Print and shaded views of the part. All mm, measured from the part's lowest x, y and z. A direction names the side the tool comes from. Coordinates: 2 decimals unless noted, no trailing zeros. Order: outer loops, then holes, each group sorted by start corner. A loop starts at its lowest first (then second) coordinate and runs counter-clockwise, first axis right, second up. Notation, with made-up numbers: M 36,77 L 65,77 A16 ccw 65,89 Z; hole C -26,19 d2. An arc over 180 degrees is marked long. One line per item, written item: value.
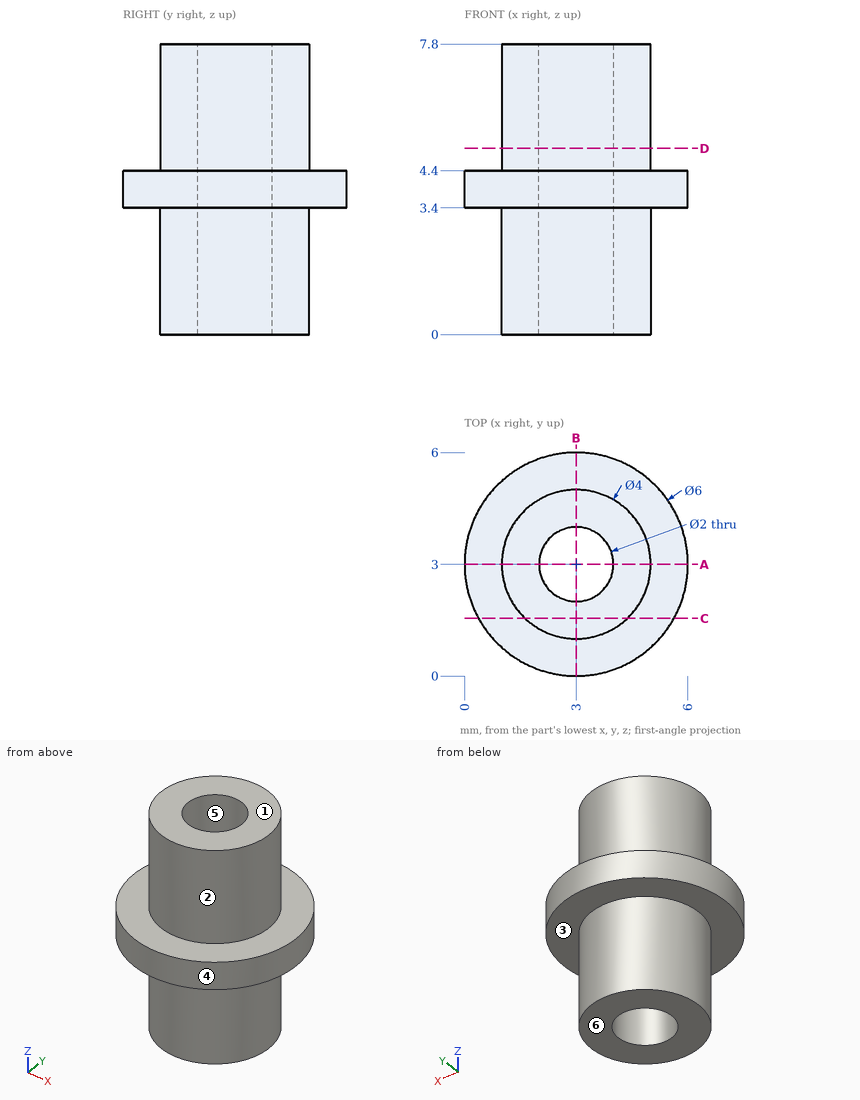
Q1. Slice it at C-C (y = 1.55). List the corners of the cut face in (x, z), plus the area to 3 significant figures.
Recorded:
outline: M 0.37,3.4 L 1.62,3.4 L 1.62,0 L 4.38,0 L 4.38,3.4 L 5.63,3.4 L 5.63,4.4 L 4.38,4.4 L 4.38,7.8 L 1.62,7.8 L 1.62,4.4 L 0.37,4.4 Z
area: 24.0 mm^2
Q2. Which spindle directions (+Z, -Z, +X, -X, +Y, -Y) get a long thin tool onto all of the face, cutting with end or side? Do the marked faces 1, 2 and 3. Say none if no direction does.
Recorded:
face 1: +Z, +X, -X, +Y, -Y
face 2: +Z
face 3: -Z
Q3. Pin check, flat tips, straight feed: pin 1 Ø2 at (y, z) = (5, 2) entering from +X; pin 2 Ø1.5 at (y, z) = (5, 4) entering from -X; pin 3 Ø2 at (y, z) = (2, 1.5) entering from -X. Stop position of each tip, or through.
Recorded:
pin 1: stops at x = 4.73
pin 2: stops at x = 0.27
pin 3: stops at x = 1
Q4. Drill centre lines: line 1 along Y through (x, z) = (3, 1.75); line 2 along Z through (x, y) = (0.35, 3.8); line 3 along X through (y, z) = (2.5, 2.75). Where is each one in solid material? Low to high.
Recorded:
line 1: y = 1 to 2, 4 to 5
line 2: z = 3.4 to 4.4
line 3: x = 1.06 to 2.13, 3.87 to 4.94
Q5. Mould opens along X. For the marked faces 4, 5 and 6 say: released by +X, released by -X, zero draft, split by the parting line, or undercut.
Recorded:
face 4: split by the parting line
face 5: undercut
face 6: zero draft
Q6. Slice it at D-D (z = 5). List the corners of the cut face in (x, y), plus the area to 3 significant figures.
Recorded:
outline: C 3,3 d4; hole C 3,3 d2
area: 9.42 mm^2
Q7. Slice it at A-A (y = 3). List the corners of the cut face in (x, z).
Recorded:
outline: M 0,3.4 L 1,3.4 L 1,0 L 2,0 L 2,7.8 L 1,7.8 L 1,4.4 L 0,4.4 Z; M 4,0 L 5,0 L 5,3.4 L 6,3.4 L 6,4.4 L 5,4.4 L 5,7.8 L 4,7.8 Z
